```python
from build123d import *

# Parameters (mm, degrees)
F0_W         = 88.9
F0_H         = 50.8
F1_DEPTH     = 177.8
F3_D         = 19.05
F5_D         = 25.4
F6_T1_DEPTH  = 167.64
F6_T3_DEPTH  = 78.74
F6_T5_DEPTH  = 40.64
F6_S9_W      = 5.08
F6_S9_H      = 5.08
F6_T10_DEPTH = 5.08
F6_S15_W     = 5.08
F6_S15_H     = 5.08
F6_T16_DEPTH = 5.08
F6_S21_W     = 5.08
F6_S21_H     = 5.08
F6_T22_DEPTH = 5.08
F6_S27_W     = 5.08
F6_S27_H     = 5.08
F6_T28_DEPTH = 5.08
F6_S33_W     = 5.08
F6_S33_H     = 5.08
F6_T34_DEPTH = 5.08
F6_S39_W     = 5.08
F6_S39_H     = 5.08
F6_T40_DEPTH = 5.08
F6_S45_W     = 5.08
F6_S45_H     = 5.08
F6_T46_DEPTH = 5.08
F6_S51_W     = 5.08
F6_S51_H     = 5.08
F6_T52_DEPTH = 5.08


# Not quite as in the source:
# - a fillet or chamfer that OpenCascade refuses, or shapes differently, is made with other operations: its cross-section is extruded or revolved along the edge and cut away or added


with BuildPart() as f1:
    # F0 (on Front) → F1 (new body)
    with BuildSketch(Plane.XZ):
        Rectangle(F0_W, F0_H)
    extrude(amount=F1_DEPTH)

    # F3 (through all)
    with Locations(Plane.XZ.offset(177.8)):
        with Locations((-30.7692382485, 0), (-6.8131890148, 0)):
            Hole(F3_D / 2)

    # F5 (through all)
    with Locations(Plane(origin=(0, 0, 0), x_dir=(1, 0, 0), z_dir=(0, 1, 0))):
        with Locations((23.0769272894, 0)):
            Hole(F5_D / 2)

    # F6: fillet of radius 5.08 on 12 edges, made by hand

    # F6_s2 → F6_t1 (cut)
    with BuildSketch(Plane.XZ.offset(5.08)):
        with BuildLine():
            ThreePointArc((44.45, 20.32), (42.9621024484, 23.9121024484), (39.37, 25.4))
            Line((39.37, 25.4), (44.45, 25.4))
            Line((44.45, 25.4), (44.45, 20.32))
        make_face()
        with BuildLine():
            ThreePointArc((-44.45, 20.32), (-42.9621024484, 23.9121024484), (-39.37, 25.4))
            Line((-39.37, 25.4), (-44.45, 25.4))
            Line((-44.45, 25.4), (-44.45, 20.32))
        make_face()
        with BuildLine():
            ThreePointArc((39.37, -25.4), (42.9621024484, -23.9121024484), (44.45, -20.32))
            Line((44.45, -20.32), (44.45, -25.4))
            Line((44.45, -25.4), (39.37, -25.4))
        make_face()
        with BuildLine():
            ThreePointArc((-39.37, -25.4), (-42.9621024484, -23.9121024484), (-44.45, -20.32))
            Line((-44.45, -20.32), (-44.45, -25.4))
            Line((-44.45, -25.4), (-39.37, -25.4))
        make_face()
    extrude(amount=F6_T1_DEPTH, mode=Mode.SUBTRACT)

    # F6_s4 → F6_t3 (cut)
    with BuildSketch(Plane.YZ.offset(-39.37)):
        with BuildLine():
            ThreePointArc((0, 20.32), (-1.4878975516, 23.9121024484), (-5.08, 25.4))
            Line((-5.08, 25.4), (0, 25.4))
            Line((0, 25.4), (0, 20.32))
        make_face()
        with BuildLine():
            ThreePointArc((-177.8, 20.32), (-176.3121024484, 23.9121024484), (-172.72, 25.4))
            Line((-172.72, 25.4), (-177.8, 25.4))
            Line((-177.8, 25.4), (-177.8, 20.32))
        make_face()
        with BuildLine():
            ThreePointArc((-5.08, -25.4), (-1.4878975516, -23.9121024484), (0, -20.32))
            Line((0, -20.32), (0, -25.4))
            Line((0, -25.4), (-5.08, -25.4))
        make_face()
        with BuildLine():
            ThreePointArc((-172.72, -25.4), (-176.3121024484, -23.9121024484), (-177.8, -20.32))
            Line((-177.8, -20.32), (-177.8, -25.4))
            Line((-177.8, -25.4), (-172.72, -25.4))
        make_face()
    extrude(amount=F6_T3_DEPTH, mode=Mode.SUBTRACT)

    # F6_s6 → F6_t5 (cut)
    with BuildSketch(Plane.XY.offset(-20.32)):
        with BuildLine():
            ThreePointArc((44.45, -5.08), (42.9621024484, -1.4878975516), (39.37, 0))
            Line((39.37, 0), (44.45, 0))
            Line((44.45, 0), (44.45, -5.08))
        make_face()
        with BuildLine():
            ThreePointArc((44.45, -172.72), (42.9621024484, -176.3121024484), (39.37, -177.8))
            Line((39.37, -177.8), (44.45, -177.8))
            Line((44.45, -177.8), (44.45, -172.72))
        make_face()
        with BuildLine():
            ThreePointArc((-44.45, -5.08), (-42.9621024484, -1.4878975516), (-39.37, 0))
            Line((-39.37, 0), (-44.45, 0))
            Line((-44.45, 0), (-44.45, -5.08))
        make_face()
        with BuildLine():
            ThreePointArc((-44.45, -172.72), (-42.9621024484, -176.3121024484), (-39.37, -177.8))
            Line((-39.37, -177.8), (-44.45, -177.8))
            Line((-44.45, -177.8), (-44.45, -172.72))
        make_face()
    extrude(amount=F6_T5_DEPTH, mode=Mode.SUBTRACT)


with BuildPart() as f6_tool8:
    # F6_s9 → F6_t10 (new body)
    with BuildSketch(Plane.YZ.offset(39.37)):
        with Locations((-2.54, 22.86)):
            Rectangle(F6_S9_W, F6_S9_H)
    extrude(amount=F6_T10_DEPTH)

    # F6_s11 → F6_t12 (revolve, cut)
    with BuildSketch(Plane(origin=(39.37, -5.08, 20.32), x_dir=(0, -0.7071067812, -0.7071067812), z_dir=(0, -0.7071067812, 0.7071067812))):
        with BuildLine():
            ThreePointArc((0, -5.08), (5.08, 0), (0, 5.08))
            Line((0, 5.08), (0, -5.08))
        make_face()
    revolve(axis=Axis((39.37, -5.08, 20.32), (1, 0, 0)), mode=Mode.SUBTRACT)


with BuildPart() as f1_1:
    add(f1.part)

    # F6_t7: cut F6_tool8
    add(f6_tool8.part, mode=Mode.SUBTRACT)


with BuildPart() as f6_tool14:
    # F6_s15 → F6_t16 (new body)
    with BuildSketch(Plane.YZ.offset(39.37)):
        with Locations((-175.26, 22.86)):
            Rectangle(F6_S15_W, F6_S15_H)
    extrude(amount=F6_T16_DEPTH)

    # F6_s17 → F6_t18 (revolve, cut)
    with BuildSketch(Plane(origin=(39.37, -172.72, 20.32), x_dir=(0, 0.7071067812, -0.7071067812), z_dir=(0, -0.7071067812, -0.7071067812))):
        with BuildLine():
            ThreePointArc((0, -5.08), (5.08, 0), (0, 5.08))
            Line((0, 5.08), (0, -5.08))
        make_face()
    revolve(axis=Axis((39.37, -172.72, 20.32), (1, 0, 0)), mode=Mode.SUBTRACT)


with BuildPart() as f1_2:
    add(f1_1.part)

    # F6_t13: cut F6_tool14
    add(f6_tool14.part, mode=Mode.SUBTRACT)


with BuildPart() as f6_tool20:
    # F6_s21 → F6_t22 (new body)
    with BuildSketch(Plane.YZ.offset(-39.37)):
        with Locations((-2.54, 22.86)):
            Rectangle(F6_S21_W, F6_S21_H)
    extrude(amount=-F6_T22_DEPTH)

    # F6_s23 → F6_t24 (revolve, cut)
    with BuildSketch(Plane(origin=(-39.37, -5.08, 20.32), x_dir=(0, -0.7071067812, -0.7071067812), z_dir=(0, 0.7071067812, -0.7071067812))):
        with BuildLine():
            ThreePointArc((0, -5.08), (5.08, 0), (0, 5.08))
            Line((0, 5.08), (0, -5.08))
        make_face()
    revolve(axis=Axis((-39.37, -5.08, 20.32), (-1, 0, 0)), mode=Mode.SUBTRACT)


with BuildPart() as f1_3:
    add(f1_2.part)

    # F6_t19: cut F6_tool20
    add(f6_tool20.part, mode=Mode.SUBTRACT)


with BuildPart() as f6_tool26:
    # F6_s27 → F6_t28 (new body)
    with BuildSketch(Plane.YZ.offset(-39.37)):
        with Locations((-175.26, 22.86)):
            Rectangle(F6_S27_W, F6_S27_H)
    extrude(amount=-F6_T28_DEPTH)

    # F6_s29 → F6_t30 (revolve, cut)
    with BuildSketch(Plane(origin=(-39.37, -172.72, 20.32), x_dir=(0, 0.7071067812, -0.7071067812), z_dir=(0, 0.7071067812, 0.7071067812))):
        with BuildLine():
            ThreePointArc((0, -5.08), (5.08, 0), (0, 5.08))
            Line((0, 5.08), (0, -5.08))
        make_face()
    revolve(axis=Axis((-39.37, -172.72, 20.32), (-1, 0, 0)), mode=Mode.SUBTRACT)


with BuildPart() as f1_4:
    add(f1_3.part)

    # F6_t25: cut F6_tool26
    add(f6_tool26.part, mode=Mode.SUBTRACT)


with BuildPart() as f6_tool32:
    # F6_s33 → F6_t34 (new body)
    with BuildSketch(Plane.XY.offset(-20.32)):
        with Locations((41.91, -2.54)):
            Rectangle(F6_S33_W, F6_S33_H)
    extrude(amount=-F6_T34_DEPTH)

    # F6_s35 → F6_t36 (revolve, cut)
    with BuildSketch(Plane(origin=(39.37, -5.08, -20.32), x_dir=(-0.7071067812, -0.7071067812, 0), z_dir=(0.7071067812, -0.7071067812, 0))):
        with BuildLine():
            ThreePointArc((0, -5.08), (5.08, 0), (0, 5.08))
            Line((0, 5.08), (0, -5.08))
        make_face()
    revolve(axis=Axis((39.37, -5.08, -20.32), (0, 0, -1)), mode=Mode.SUBTRACT)


with BuildPart() as f1_5:
    add(f1_4.part)

    # F6_t31: cut F6_tool32
    add(f6_tool32.part, mode=Mode.SUBTRACT)


with BuildPart() as f6_tool38:
    # F6_s39 → F6_t40 (new body)
    with BuildSketch(Plane.XY.offset(-20.32)):
        with Locations((41.91, -175.26)):
            Rectangle(F6_S39_W, F6_S39_H)
    extrude(amount=-F6_T40_DEPTH)

    # F6_s41 → F6_t42 (revolve, cut)
    with BuildSketch(Plane(origin=(39.37, -172.72, -20.32), x_dir=(-0.7071067812, 0.7071067812, 0), z_dir=(-0.7071067812, -0.7071067812, 0))):
        with BuildLine():
            ThreePointArc((0, -5.08), (5.08, 0), (0, 5.08))
            Line((0, 5.08), (0, -5.08))
        make_face()
    revolve(axis=Axis((39.37, -172.72, -20.32), (0, 0, -1)), mode=Mode.SUBTRACT)


with BuildPart() as f1_6:
    add(f1_5.part)

    # F6_t37: cut F6_tool38
    add(f6_tool38.part, mode=Mode.SUBTRACT)


with BuildPart() as f6_tool44:
    # F6_s45 → F6_t46 (new body)
    with BuildSketch(Plane.XY.offset(-20.32)):
        with Locations((-41.91, -2.54)):
            Rectangle(F6_S45_W, F6_S45_H)
    extrude(amount=-F6_T46_DEPTH)

    # F6_s47 → F6_t48 (revolve, cut)
    with BuildSketch(Plane(origin=(-39.37, -5.08, -20.32), x_dir=(0.7071067812, -0.7071067812, 0), z_dir=(0.7071067812, 0.7071067812, 0))):
        with BuildLine():
            ThreePointArc((0, -5.08), (5.08, 0), (0, 5.08))
            Line((0, 5.08), (0, -5.08))
        make_face()
    revolve(axis=Axis((-39.37, -5.08, -20.32), (0, 0, -1)), mode=Mode.SUBTRACT)


with BuildPart() as f1_7:
    add(f1_6.part)

    # F6_t43: cut F6_tool44
    add(f6_tool44.part, mode=Mode.SUBTRACT)


with BuildPart() as f6_tool50:
    # F6_s51 → F6_t52 (new body)
    with BuildSketch(Plane.XY.offset(-20.32)):
        with Locations((-41.91, -175.26)):
            Rectangle(F6_S51_W, F6_S51_H)
    extrude(amount=-F6_T52_DEPTH)

    # F6_s53 → F6_t54 (revolve, cut)
    with BuildSketch(Plane(origin=(-39.37, -172.72, -20.32), x_dir=(0.7071067812, 0.7071067812, 0), z_dir=(-0.7071067812, 0.7071067812, 0))):
        with BuildLine():
            ThreePointArc((0, -5.08), (5.08, 0), (0, 5.08))
            Line((0, 5.08), (0, -5.08))
        make_face()
    revolve(axis=Axis((-39.37, -172.72, -20.32), (0, 0, -1)), mode=Mode.SUBTRACT)


with BuildPart() as f1_8:
    add(f1_7.part)

    # F6_t49: cut F6_tool50
    add(f6_tool50.part, mode=Mode.SUBTRACT)


solid = f1_8.part
```
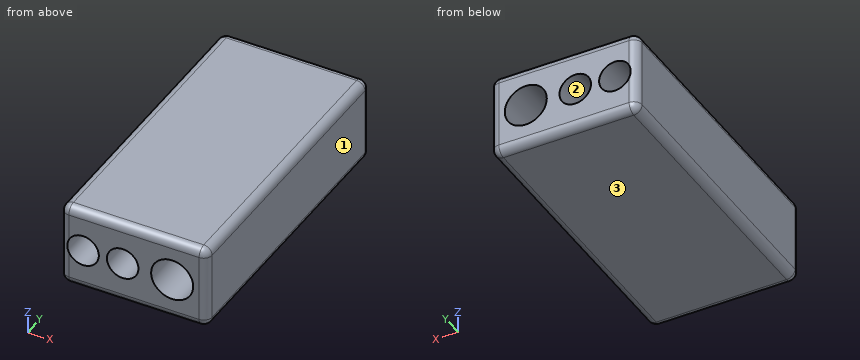
Read the model definition and answer for the solid it produces. Units are mm, in the model's axes. Face numbers are marked on the shaded views. Coordinates: 2 decimals unless noted, no trailing zeros. Write each loop counter-clockwise with the first axis right and the second up, starting at its lowest first coordinate (ties: lowest second). Pieces come first, ordered by that corner, then holes. Notation, with made-up numbers: (41, 58) - (82, 58) arc R23 cw to (82, 75) - close; hole circle Ø3 at (76, 60.25). An arc over 180 degrees is marked (long way). Answer as a JSON object with one key per item and string values. Group by question number.
1. Consider L1, parallel to X at y = -167, z = 1.5; L2, parallel to X at y = -88.5, z = 5.5; L3, parallel to Z at x = 27, y = -39.5. Determine where each line is inside the solid, lowest interval first. Write a range as [from, to].
2. A cutting plane is placed at D-D (x = -7). Determine the outline of the cut face in (y, z), plus the area to 3 significant figures.
3. The mould has two halves that part along X. Classify the marked faces 1, 2 and 3: +X half, -X half, draft (parallel to the pull), parting line (faces both ways), or undercut.
4. A cutting plane is placed at C-C (z = 0). Determine the outline of the cut face in (x, y).
5. A cutting plane is placed at B-B (x = -37.5). Determine the outline of the cut face in (y, z), plus the area to 3 significant figures.
6. A cutting plane is placed at A-A (y = -65). Determine the outline of the cut face in (x, z) (3 decimals).
Worked out:
{
 "1": {"L1": "x = [-44.45, -40.18], [-21.36, -16.22], [2.59, 10.47], [35.69, 44.45]", "L2": "x = [-44.45, -38.55], [-22.99, -14.59], [0.96, 11.63], [34.52, 44.45]", "L3": "z = [-25.4, -12.08], [12.08, 25.4]"},
 "2": {"outline": "(-177.8, -20.32) arc R5.08 ccw to (-172.72, -25.4) - (-5.08, -25.4) arc R5.08 ccw to (0, -20.32) - (0, -9.52) - (-177.8, -9.52) - close; (-177.8, 9.52) - (0, 9.52) - (0, 20.32) arc R5.08 ccw to (-5.08, 25.4) - (-172.72, 25.4) arc R5.08 ccw to (-177.8, 20.32) - close", "area": "5,620 mm²"},
 "3": {"face 1": "+X half", "face 2": "undercut", "face 3": "draft"},
 "4": {"outline": "(-44.45, -172.72) arc R5.08 ccw to (-40.29, -177.72) - (-40.29, -0.08) arc R5.08 ccw to (-44.45, -5.08) - close; (-21.24, -177.8) - (-16.34, -177.8) - (-16.34, 0) - (-21.24, 0) - close; (2.71, -177.8) - (10.38, -177.8) - (10.38, 0) - (2.71, 0) - close; (35.78, -177.8) - (39.37, -177.8) arc R5.08 ccw to (44.45, -172.72) - (44.45, -5.08) arc R5.08 ccw to (39.37, 0) - (35.78, 0) - close"},
 "5": {"outline": "(-177.8, -20.32) arc R5.08 ccw to (-172.72, -25.4) - (-5.08, -25.4) arc R5.08 ccw to (0, -20.32) - (0, -6.74) - (-177.8, -6.74) - close; (-177.8, 6.74) - (0, 6.74) - (0, 20.32) arc R5.08 ccw to (-5.08, 25.4) - (-172.72, 25.4) arc R5.08 ccw to (-177.8, 20.32) - close", "area": "6,610 mm²"},
 "6": {"outline": "(-44.45, -20.32) arc R5.08 ccw to (-39.37, -25.4) - (39.37, -25.4) arc R5.08 ccw to (44.45, -20.32) - (44.45, 20.32) arc R5.08 ccw to (39.37, 25.4) - (-39.37, 25.4) arc R5.08 ccw to (-44.45, 20.32) - close; hole circle Ø19.05 at (-30.769, 0); hole circle Ø19.05 at (-6.813, 0); hole circle Ø25.4 at (23.077, 0)"}
}
